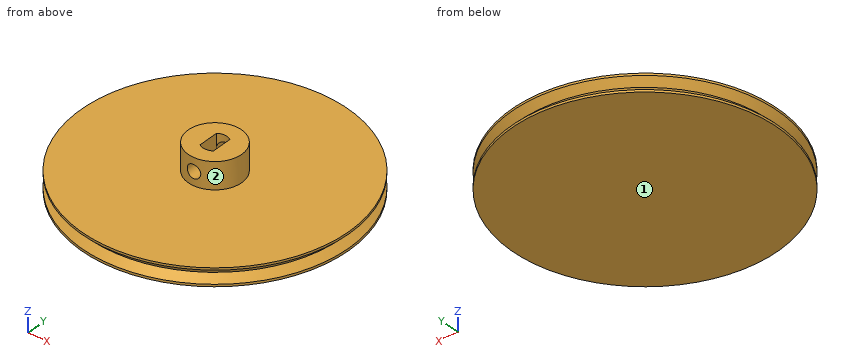
```python
from build123d import *

# Parameters (mm, degrees)
F0_R     = 30
F0_R_2   = 6
F1_DEPTH = 4
F2_DEPTH = 6
F3_R     = 1.5
F4_DEPTH = 12.5
F5_W     = 3
F5_H     = 4.6
F6_DEPTH = 9.4


with BuildPart() as f1:
    # F0 (on Top) → F1 (new body)
    with BuildSketch(Plane.XY):
        Circle(F0_R)
        Circle(F0_R_2, mode=Mode.SUBTRACT)
        Circle(F0_R_2)
    extrude(amount=-F1_DEPTH)

    # F0 (on Top) → F2 (join)
    with BuildSketch(Plane.XY):
        Circle(F0_R_2)
    extrude(amount=F2_DEPTH)

    # F3 (on Front) → F4 (cut, symmetric)
    with BuildSketch(Plane.XZ):
        with Locations((0, 3)):
            Circle(F3_R)
    extrude(amount=F4_DEPTH, both=True, mode=Mode.SUBTRACT)

    # F5 (on face) → F6 (cut)
    with BuildSketch(Plane.XY.offset(6)):
        with BuildLine():
            ThreePointArc((1.5, 2.3), (0, 2.747197), (-1.5, 2.3))
            Line((-1.5, 2.3), (1.5, 2.3))
        make_face()
        Rectangle(F5_W, F5_H)
        with BuildLine():
            Line((1.5, -2.3), (-1.5, -2.3))
            ThreePointArc((-1.5, -2.3), (0, -2.752803), (1.5, -2.3))
        make_face()
    extrude(amount=-F6_DEPTH, mode=Mode.SUBTRACT)

    # F7 (on Front) → F8 (revolve, cut)
    with BuildSketch(Plane.XZ):
        Polygon((30, -3.483821), (30, -0.483821), (28.5, -1.983821), align=None)
    revolve(axis=Axis((0, 0, -0.420868), (0, 0, -1)), mode=Mode.SUBTRACT)


solid = f1.part
```
CAD build for the part. Positions are in the model's coordinates, mm. Face numbers are marked on the shaded views. A direction names the side the tool comes from. Round coordinates to 2 decimals unless told otherwise and drop trailing zeros. Write each loop counter-clockwise with the first axis right and the second up, starting at its lowest first coordinate (ties: lowest second). Pieces come first, ordered by that corner, then holes. Notation, with made-up numbers: (-3, 8) -> (45, 8) arc R14 cw to (45, 14) -> close; hole circle Ø5 at (-9, 71). An arc over 180 degrees is marked (long way). Answer in a Markdown table with one row per item. Add a question column.
Item 1: Saw through at B-B, the plane y = 0. Write the cut outline in (x, z), then the cut area to 3 significant figures.
Item 2: Drop flat-ended pins along their axis: pin 1 Ø1.5 at (y, z) = (16.5, 2.5) entering from -X; pin 2 Ø0.9 at (x, y) = (0, 1) entering from +Z; pin 3 Ø5 at (x, y) = (-23, -8.5) entering from +Z. Give the stop position or say it passes through.
Item 3: Drill centre lines: line 1 (Z direction, x = 0, y = 4); line 2 (Z direction, x = -11.5, y = -2.5); line 3 (X direction, y = -4.1, z = 3). Where is each one in solid material? Low to high. Write a range as from..to.
Item 4: Saw through at A-A, the plane x = 0. Write the cut outline in (y, z).
Item 5: Which spindle directions (+Z, -Z, +X, -X, +Y, -Y) get a long thin tool onto all of the face, cutting with end or side? Do the marked faces 1 and 2. Say none if no direction does.
Findings below:
| question | item | result |
|---|---|---|
| 1 | outline | (-30, -4) -> (30, -4) -> (30, -3.48) -> (28.5, -1.98) -> (30, -0.48) -> (30, 0) -> (6, 0) -> (6, 6) -> (1.5, 6) -> (1.5, -3.4) -> (-1.5, -3.4) -> (-1.5, 6) -> (-6, 6) -> (-6, 0) -> (-30, 0) -> (-30, -0.48) -> (-28.5, -1.98) -> (-30, -3.48) -> close |
| 1 | area | 279 mm^2 |
| 2 | pin 1 | passes through |
| 2 | pin 2 | stops at z = -3.4 |
| 2 | pin 3 | stops at z = 0 |
| 3 | line 1 | z = -4..1.5, 4.5..6 |
| 3 | line 2 | z = -4..0 |
| 3 | line 3 | x = -4.38..-1.5, 1.5..4.38 |
| 4 | outline | (-30, -4) -> (30, -4) -> (30, -3.48) -> (28.5, -1.98) -> (30, -0.48) -> (30, 0) -> (6, 0) -> (6, 1.5) -> (2.75, 1.5) -> (2.75, -3.4) -> (-2.75, -3.4) -> (-2.75, 1.5) -> (-6, 1.5) -> (-6, 0) -> (-30, 0) -> (-30, -0.48) -> (-28.5, -1.98) -> (-30, -3.48) -> close; (-6, 4.5) -> (-2.75, 4.5) -> (-2.75, 6) -> (-6, 6) -> close; (2.75, 4.5) -> (6, 4.5) -> (6, 6) -> (2.75, 6) -> close |
| 5 | face 1 | -Z, +X, -X, +Y, -Y |
| 5 | face 2 | +Z |
